Part model, mm, in its own coordinate system. A direction names the side the tool comes from. Give positions to 0.01 mm unless a question says otherwise; leave off trailing zeros. Order: outer loops, then holes, each group sorted by start corner. A loop starts at its lowest first (then second) coordinate and runs counter-clockwise, first axis right, second up. Notation, with made-up numbers: M 77,68 L 111,68 A14 cw 111,82 Z; hole C 4.5,-4.5 d5. An arc over 180 degrees is marked long. Answer as a JSON object with one key per item and string values.
Autodesk Fusion 360 part; units mm, degrees
sketch "Base" plane through (0, 0, 0) normal (0, 0, 1) x (1, 0, 0)
  circle A0 centre (0, 0) radius 17.5
  circle A1 centre (-15, 0) radius 2
  circle A2 centre (15, 0) radius 2
  line L0 (0.5638, -7.0807) -> (0.5638, 7.0807)
  arc A3 (0.5638, 7.0807) -> (-4.4362, 7.0807) centre (-1.9362, 7.0807) ccw
  line L1 (-4.4362, 7.0807) -> (-4.4362, -7.0807)
  arc A4 (-4.4362, -7.0807) -> (0.5638, -7.0807) centre (-1.9362, -7.0807) ccw
  line L2 (-1.9362, -7.0807) -> (-1.9362, 7.0807) construction
  point P0 (-1.9362, 0)
  dimension "d1" = 35
  dimension "d2" = 4
  dimension "d3" = 4
  dimension "d4" = 15
  dimension "d5" = 15
  dimension "d6" = 5
extrude "Extrude1" add sketch "Base" along normal blind 4
sketch "Board Bed" plane through (0, 0, 4) normal (0, 0, 1) x (1, 0, 0)
  line L0 (-9.4362, 13) -> (-7.4362, 13)
  line L1 (-7.4362, 13) -> (-7.4362, -13)
  line L2 (-7.4362, -13) -> (-9.4362, -13)
  line L3 (-9.4362, -13) -> (-9.4362, 13)
  circle A0 centre (-15, 0) radius 2
  arc A1 (-4.4362, -7.0807) -> (0.5638, -7.0807) centre (-1.9362, -7.0807) ccw
  line L4 (-4.4362, -7.0807) -> (-4.4362, 7.0807)
  arc A2 (0.5638, 7.0807) -> (-4.4362, 7.0807) centre (-1.9362, 7.0807) ccw
  line L5 (0.5638, 7.0807) -> (0.5638, -7.0807)
  circle A3 centre (15, 0) radius 2
  circle A4 centre (0, 0) radius 17.5
  dimension "d9" = 26
  dimension "d10" = 13
  dimension "d13" = 3
extrude "Extrude2" add sketch "Board Bed" along normal blind 65 contours L0 L1 L2 L3
sketch "Sketch4" plane through (-7.4362, 0, 0) normal (1, 0, 0) x (0, 1, 0)
  line L0 (-13, 4) -> (13, 4)
  line L1 (13, 4) -> (13, 69)
  line L2 (13, 69) -> (-13, 69)
  line L3 (-13, 69) -> (-13, 4)
  circle A0 centre (7.62, 6.58) radius 1.25
  circle A1 centre (-7.62, 6.58) radius 1.25
  circle A2 centre (-10.16, 65) radius 1.25
  circle A3 centre (10.16, 65) radius 1.25
  dimension "d14" = 2.5
  dimension "d15" = 2.5
  dimension "d16" = 15.24
  dimension "d17" = 7.62
  dimension "d18" = 2.5
  dimension "d19" = 2.5
  dimension "d20" = 10.16
  dimension "d21" = 10.16
  dimension "d22" = 20.32
  dimension "d25" = 58.42
  dimension "d26" = 58.42
  dimension "d28" = 2.58
  dimension "d29" = 2.58
extrude "Extrude3" cut sketch "Sketch4" against normal blind 5 contours A0 | A1 | A2 | A3
1. Pin check, flat tips, straight feed: P1, Ø12, axis at x = -4, z = 27, coming from the +Y side; P2, Ø10, axis at y = 12, z = 15, coming from the -X side; P3, Ø1.5, axis at y = 5, z = 19.5, coming from the +X side. Stop position of each tip, or through.
Worked answers:
{"P1": "stops at y = 13", "P2": "stops at x = -9.44", "P3": "stops at x = -7.44"}
2. Cut at A-A on z = 65. Give the cut face in (x, y), plus the area to 3 significant figures.
Worked answers:
{"outline": "M -9.44,-13 L -7.44,-13 L -7.44,-11.41 L -9.44,-11.41 Z; M -9.44,-8.91 L -7.44,-8.91 L -7.44,8.91 L -9.44,8.91 Z; M -9.44,11.41 L -7.44,11.41 L -7.44,13 L -9.44,13 Z", "area": "42.0 mm^2"}
3. Cut at C-C on x = 4.5. Give the cut face in (y, z), plus the area to 3 significant figures.
Worked answers:
{"outline": "M -16.91,0 L 16.91,0 L 16.91,4 L -16.91,4 Z", "area": "135 mm^2"}
4. Cut at D-D on x = 12. Give the cut face in (y, z).
Worked answers:
{"outline": "M -12.74,0 L 12.74,0 L 12.74,4 L -12.74,4 Z"}
5. Which spindle directions (+Z, -Z, +X, -X, +Y, -Y) get a long thin tool onto all of the face, cutting with end or side? Do faces 4 (the flat face through (-7.436, 0, 36)), 5 (the flat face through (0.564, 0, 2)), 6 (the flat face through (-9.436, 0, 36)), 7 (the flat face through (4, 0, 0)), 8 (the flat face through (-8, 13, 36)). Say none if no direction does.
Worked answers:
{"face 4": "+Z, +X, +Y, -Y", "face 5": "+Z, -Z", "face 6": "+Z, -X, +Y, -Y", "face 7": "-Z, +X, -X, +Y, -Y", "face 8": "+Z, +X, -X, +Y"}
6. Two-plate mould, pull along Y, no slides. Class faces 1 (the flat face through (-8, -13, 36)), 2 (the cylindrical face through (13.4, 1.2, 2)), 3 (the cylindrical face through (-13.887, 10.648, 1.972)): +Y half, -Y half, draft (parallel to the pull), parting line (faces both ways), or undercut.
Worked answers:
{"face 1": "-Y half", "face 2": "undercut", "face 3": "parting line"}
7. Cut at B-B on y = 0. Give the cut face in (x, z).
Worked answers:
{"outline": "M -17.5,0 L -17,0 L -17,4 L -17.5,4 Z; M -13,0 L -4.44,0 L -4.44,4 L -7.44,4 L -7.44,69 L -9.44,69 L -9.44,4 L -13,4 Z; M 0.56,0 L 13,0 L 13,4 L 0.56,4 Z; M 17,0 L 17.5,0 L 17.5,4 L 17,4 Z"}
8. Probe line 1 along Y through (x, z) = (-8, 65); line 2 along Z through (x, y) = (-8.15, -10.16); line 3 along X through (y, z) = (-4, 14.5). List the from-to ranges inside material, lowest first.
Worked answers:
{"line 1": "y = -13 to -11.41, -8.91 to 8.91, 11.41 to 13", "line 2": "z = 0 to 63.75, 66.25 to 69", "line 3": "x = -9.44 to -7.44"}
